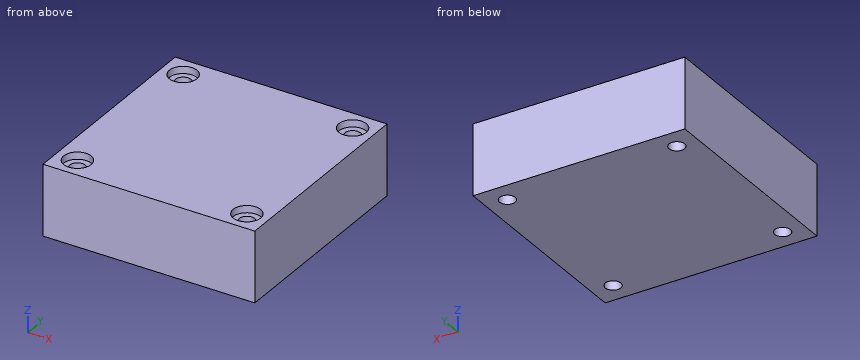
```python
from build123d import *

# Parameters (mm, degrees)
SKETCH2_W                                       = 76.2
SKETCH2_H                                       = 76.2
BOSS_EXTRUDE1_DEPTH                             = 25.4
CBORE_FOR_10_BUTTON_HEAD_CAP_SCREW1_D           = 5.6134
CBORE_FOR_10_BUTTON_HEAD_CAP_SCREW1_CBORE_D     = 9.92124
CBORE_FOR_10_BUTTON_HEAD_CAP_SCREW1_CBORE_DEPTH = 2.5654


with BuildPart() as part:
    # Sketch2 → Boss-Extrude1 (new body)
    with BuildSketch(Plane.XY):
        with Locations((38.1, 38.1)):
            Rectangle(SKETCH2_W, SKETCH2_H)
    extrude(amount=BOSS_EXTRUDE1_DEPTH)

    # CBORE for #10 Button Head Cap Screw1 (through all)
    with Locations(Plane.XY.offset(25.4)):
        with Locations((7.62, 68.58), (68.58, 68.58), (68.58, 7.62), (7.62, 7.62)):
            CounterBoreHole(CBORE_FOR_10_BUTTON_HEAD_CAP_SCREW1_D / 2, CBORE_FOR_10_BUTTON_HEAD_CAP_SCREW1_CBORE_D / 2, CBORE_FOR_10_BUTTON_HEAD_CAP_SCREW1_CBORE_DEPTH)


solid = part.part
```
Could you check a few things on this model? Use its own coordinates, in mm. Coordinates: 2 decimals unless noted, no trailing zeros. Write each loop counter-clockwise with the first axis right and the second up, starting at its lowest first coordinate (ties: lowest second). Pieces come first, ordered by that corner, then holes. Notation, with made-up numbers: (47.5, 33) - (91.5, 33) arc R15 ccw to (91.5, 45) - close; hole circle Ø3 at (57.25, 88). An arc over 180 degrees is marked (long way). Use a Markdown table: item, result.
Q1. I'm going to push a flat-ended pin straight in: pin 1 Ø8 at (x, y) = (68.58, 7.62) entering from +Z. Where does the tip first touch, or does it pass through?
Geometry check:
| item | result |
|---|---|
| pin 1 | stops at z = 22.83 |
Q2. Imagine slicing it at C-C (z = 19.25). List the corners of the cut face in (x, y) for me, and give its area (3 significant figures).
Geometry check:
| item | result |
|---|---|
| outline | (0, 0) - (76.2, 0) - (76.2, 76.2) - (0, 76.2) - close; hole circle Ø5.61 at (7.62, 7.62); hole circle Ø5.61 at (7.62, 68.58); hole circle Ø5.61 at (68.58, 7.62); hole circle Ø5.61 at (68.58, 68.58) |
| area | 5,710 mm2 |
Q3. Imagine slicing it at A-A (x = 68.58). List the corners of the cut face in (y, z) for me.
Geometry check:
| item | result |
|---|---|
| outline | (0, 0) - (4.81, 0) - (4.81, 22.83) - (2.66, 22.83) - (2.66, 25.4) - (0, 25.4) - close; (10.43, 0) - (65.77, 0) - (65.77, 22.83) - (63.62, 22.83) - (63.62, 25.4) - (12.58, 25.4) - (12.58, 22.83) - (10.43, 22.83) - close; (71.39, 0) - (76.2, 0) - (76.2, 25.4) - (73.54, 25.4) - (73.54, 22.83) - (71.39, 22.83) - close |
Q4. Please list where these lines run through material, in increasing order: L1, parallel to Y at x = 7.62, z = 16; L2, parallel to Y at x = 68.58, z = 23.8; L3, parallel to X at y = 70, z = 17.5.
Geometry check:
| item | result |
|---|---|
| L1 | y = 0 to 4.81, 10.43 to 65.77, 71.39 to 76.2 |
| L2 | y = 0 to 2.66, 12.58 to 63.62, 73.54 to 76.2 |
| L3 | x = 0 to 5.2, 10.04 to 66.16, 71 to 76.2 |
